Design review of the part shown in the three views and the two pictorial views. Dimensions are in mm from the part's minimum x, y and z. A direction names the side the tool comes from. Give positions to 0.01 mm unless a question says otherwise; leave off trailing zeros. Order: outer loops, then holes, each group sorted by start corner. A loop starts at its lowest first (then second) coordinate and runs counter-clockwise, first axis right, second up. Notation, with made-up numbers: (19.25, 65) - (29.25, 65) arc R15 cw to (29.25, 84) - close; hole circle Ø5 at (42, -15.75). An arc over 180 degrees is marked (long way). Put each result on its own line as item: value.
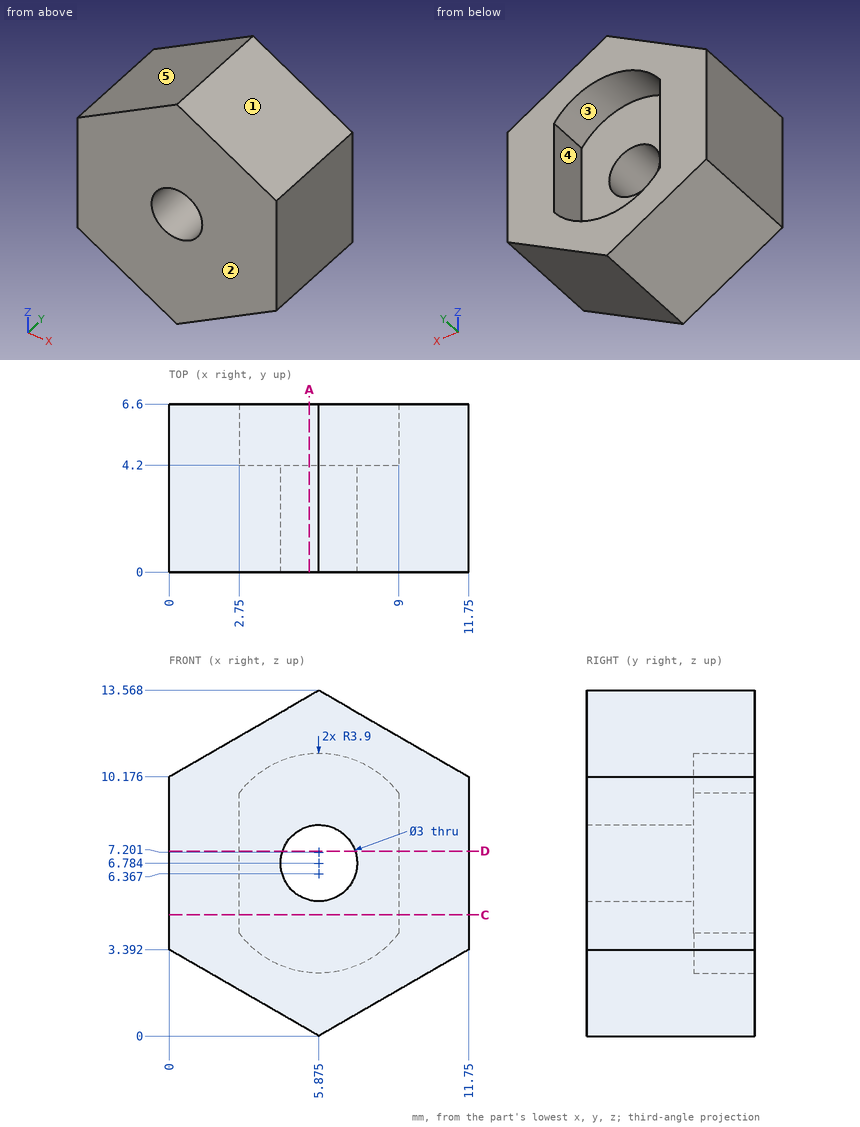
(1) Wall thickness on L1, parallel to X at y = 5, z = 6; L2, parallel to Y at x = 3.75, z = 4; L3, parallel to X at y = 5.75, z = 3.5: over which ranges is each line inside the solid? List them lowest first.
The answers:
L1: 0 to 2.75, 9 to 11.75
L2: 0 to 4.2
L3: 0 to 3.23, 8.52 to 11.75
(2) Take a section at D-D, the plane z = 7.25. Write out the cut boundary in (x, y).
The answers:
outline: (0, 0) - (4.45, 0) - (4.45, 4.2) - (2.75, 4.2) - (2.75, 6.6) - (0, 6.6) - close; (7.3, 0) - (11.75, 0) - (11.75, 6.6) - (9, 6.6) - (9, 4.2) - (7.3, 4.2) - close
(3) For the marked faces 4 and 5, list the 3-axis set-ups (+Z, -Z, +X, -X, +Y, -Y) from which the entire face can be reached by the end or side of a thin tool; tool diameter is ignored.
The answers:
face 4: +Y
face 5: +Z, -X, +Y, -Y
(4) The part is to be moulded in two halves that separate along Z. For the marked faces 1, 2 and 3, say which applies: pulls with the +Z half, pulls with the -Z half, needs draft (parallel to the pull), parting line crosses it, or undercut.
The answers:
face 1: pulls with the +Z half
face 2: needs draft
face 3: undercut
(5) Take a section at C-C, the plane z = 4.75. Write out the cut boundary in (x, y).
The answers:
outline: (0, 0) - (11.75, 0) - (11.75, 6.6) - (9, 6.6) - (9, 4.2) - (2.75, 4.2) - (2.75, 6.6) - (0, 6.6) - close
(6) Take a section at A-A, the plane x = 5.5. Write out the cut boundary in (y, z) (1 decimal).
The answers:
outline: (0, 0.2) - (6.6, 0.2) - (6.6, 2.5) - (4.2, 2.5) - (4.2, 5.3) - (0, 5.3) - close; (0, 8.2) - (4.2, 8.2) - (4.2, 11.1) - (6.6, 11.1) - (6.6, 13.4) - (0, 13.4) - close
